Part model, mm, in its own coordinate system. Round coordinates to 2 decimals unless told otherwise and drop trailing zeros. Write each loop counter-clockwise with the first axis right and the second up, starting at its lowest first coordinate (ties: lowest second). Pieces come first, ordered by that corner, then holes. Notation, with made-up numbers: M 76,53 L 126,53 A24 ccw 126,83 Z; hole C 45,81.5 d6. An arc over 180 degrees is marked long. Answer as a JSON object with one key per item and string values. Group by question number.
1. Drill centre lines: line 1 (X direction, y = 114, z = 8); line 2 (X direction, y = 129.5, z = 16.25); line 3 (X direction, y = 114.5, z = 4). Where is each one in solid material? Low to high. Write a range as from..to.
2. Two-plate mould, pull along X, no slides. Class faces 1 (the face through (439.557, 131, 9)), 2 (the face through (174.43, 158.95, 9.02)), 3 (the face through (53, 134, 0)): +X half, -X half, draft (parallel to the pull), parting line (faces both ways), or undercut.
3. Band-saw the part on B-B, the plane z = 8. Write the cut outline in (x, y) (1 decimal), plus the area to 3 significant figures.
4. Band-saw the part on A-A, the plane x = 131. Write the cut outline in (y, z), plus the area to 3 significant figures.
from build123d import *

# Parameters (mm, degrees)
SKETCH1_W           = 762
SKETCH1_H           = 203.2
BOSS_EXTRUDE1_DEPTH = 18.288
SKETCH2_R           = 14.2875
CUT_EXTRUDE1_DEPTH  = 499.404705003
SKETCH3_R           = 14.2875
CUT_EXTRUDE2_DEPTH  = 499.404705003


with BuildPart() as part:
    # Sketch1 → Boss-Extrude1 (new body)
    with BuildSketch(Plane.XY):
        with Locations((58.556886228, 132.62754491)):
            Rectangle(SKETCH1_W, SKETCH1_H)
    extrude(amount=BOSS_EXTRUDE1_DEPTH)

    # Sketch2 → Cut-Extrude1 (cut, through all)
    with BuildSketch(Plane(origin=(0, 0, 0), x_dir=(-1, 0, 0), z_dir=(0, 0, -1))):
        with Locations((112.893113772, 132.62754491)):
            Circle(SKETCH2_R)
    extrude(amount=-CUT_EXTRUDE1_DEPTH, mode=Mode.SUBTRACT)

    # Sketch3 → Cut-Extrude2 (cut, through all)
    with BuildSketch(Plane(origin=(0, 0, 0), x_dir=(-1, 0, 0), z_dir=(0, 0, -1))):
        with Locations((-128.406886228, 126.576648332)):
            Circle(SKETCH3_R)
        with Locations((-191.906886228, 126.576648332)):
            Circle(SKETCH3_R)
        with Locations((-160.156886228, 158.326648332)):
            Circle(SKETCH3_R)
        with Locations((-160.156886228, 94.826648332)):
            Circle(SKETCH3_R)
        with Locations((-7.756886228, 126.576648332)):
            Circle(SKETCH3_R)
    extrude(amount=-CUT_EXTRUDE2_DEPTH, mode=Mode.SUBTRACT)


solid = part.part
Worked answers:
{
 "1": {"line 1": "x = -322.44..0.98, 14.54..121.63, 135.19..185.13, 198.69..439.56", "line 2": "x = -322.44..-126.83, -98.95..-6.23, 21.74..114.42, 142.39..177.92, 205.89..439.56", "line 3": "x = -322.44..0.12, 15.39..120.77, 136.04..184.27, 199.54..439.56"},
 "2": {"face 1": "+X half", "face 2": "undercut", "face 3": "draft"},
 "3": {"outline": "M -322.4,31 L 439.6,31 L 439.6,234.2 L -322.4,234.2 Z; hole C -112.9,132.6 d28.6; hole C 7.8,126.6 d28.6; hole C 128.4,126.6 d28.6; hole C 160.2,94.8 d28.6; hole C 160.2,158.3 d28.6; hole C 191.9,126.6 d28.6", "area": "151,000 mm^2"},
 "4": {"outline": "M 31.03,0 L 112.53,0 L 112.53,18.29 L 31.03,18.29 Z; M 140.63,0 L 234.23,0 L 234.23,18.29 L 140.63,18.29 Z", "area": "3,200 mm^2"}
}
